Design review of the part built by this model. Coordinates are the model's own, in mm. Face numbers are marked on the shaded views. A direction names the side the tool comes from. Coordinates: 2 decimals unless noted, no trailing zeros. Write each loop counter-clockwise with the first axis right and the second up, starting at its lowest first coordinate (ties: lowest second). Pieces come first, ordered by that corner, then holes. Notation, with made-up numbers: M -16,-13 L 22,-13 A24 ccw 22,-3 Z; hole C 84.5,-9 d9. An arc over 180 degrees is marked long. One line per question, with ' | ' between items.
from build123d import *

# Parameters (mm, degrees)
F1_DEPTH = 2.8
F2_R     = 0.55
F3_DEPTH = 5
F4_R     = 1
F5_R     = 0.3
F7_W     = 2.5907744158
F7_H     = 2.3
F8_DEPTH = 1.5
F9_R     = 0.5


with BuildPart() as f1:
    # F0 (on Top) → F1 (new body)
    with BuildSketch(Plane.XY):
        with BuildLine():
            Line((-4.2, -2.5), (-3.2, -2.5))
            Line((-3.2, -2.5), (-3.2, -1.9))
            ThreePointArc((-3.2, -1.9), (-2.9071067812, -1.1928932188), (-2.2, -0.9))
            Line((-2.2, -0.9), (0, -0.9))
            Line((0, -0.9), (0, -2.3))
            Line((0, -2.3), (1.8, -2.3))
            Line((1.8, -2.3), (1.8, -1.3))
            Line((1.8, -1.3), (5.2, -1.3))
            Line((5.2, -1.3), (5.2, 0))
            Line((5.2, 0), (5.2, 1.3))
            Line((5.2, 1.3), (1.8, 1.3))
            Line((1.8, 1.3), (1.8, 2.3))
            Line((1.8, 2.3), (0, 2.3))
            Line((0, 2.3), (0, 0.9))
            Line((0, 0.9), (-2.2, 0.9))
            ThreePointArc((-2.2, 0.9), (-2.9071067812, 1.1928932188), (-3.2, 1.9))
            Line((-3.2, 1.9), (-3.2, 2.5))
            Line((-3.2, 2.5), (-4.2, 2.5))
            Line((-4.2, 2.5), (-4.6408174518, 0))
            Line((-4.6408174518, 0), (-4.2, -2.5))
        make_face()
    extrude(amount=F1_DEPTH)

    # F2 (on face) → F3 (join)
    with BuildSketch(Plane(origin=(0, 0, 0), x_dir=(1, 0, 0), z_dir=(0, 0, -1))):
        with BuildLine():
            Line((-4.2, -2.5), (-3.2, -2.5))
            Line((-3.2, -2.5), (-3.2, -1.9))
            ThreePointArc((-3.2, -1.9), (-2.9071067812, -1.1928932188), (-2.2, -0.9))
            Line((-2.2, -0.9), (-2.2, 0.9))
            ThreePointArc((-2.2, 0.9), (-2.9071067812, 1.1928932188), (-3.2, 1.9))
            Line((-3.2, 1.9), (-3.2, 2.5))
            Line((-3.2, 2.5), (-4.2, 2.5))
            Line((-4.2, 2.5), (-4.6408174518, 0))
            Line((-4.6408174518, 0), (-4.2, -2.5))
        make_face()
        with Locations((-3.6, 0)):
            Circle(F2_R, mode=Mode.SUBTRACT)
    extrude(amount=F3_DEPTH)

    # F4
    f4_edges = [f1.edges().sort_by_distance(p)[0] for p in [
        (-2.2, 0, 0),
        (-4.640817, 0, -1.1),
    ]]
    fillet(f4_edges, radius=F4_R)

    # F5
    f5_edges = [f1.edges().sort_by_distance(p)[0] for p in [
        (5.2, -1.3, 1.4),
        (5.2, 1.3, 1.4),
        (-3.2, 2.5, -1.1),
        (-4.2, 2.5, -1.1),
        (-3.2, -2.5, -1.1),
        (-4.2, -2.5, -1.1),
        (-0.6, 0.9, 0),
        (-1.2, 0, 0),
        (0, 1.6, 0),
        (-0.6, -0.9, 0),
        (0.9, 2.3, 0),
        (0, -1.6, 0),
        (1.8, 1.8, 0),
        (0.9, -2.3, 0),
        (3.5, 1.3, 0),
        (1.8, -1.8, 0),
        (5.2, 0, 0),
        (3.5, -1.3, 0),
    ]]
    fillet(f5_edges, radius=F5_R)

    # F7 (on offset) → F8 (cut)
    with BuildSketch(Plane.XY.offset(-3.2)):
        with Locations((-3.6953872079, 0)):
            Rectangle(F7_W, F7_H)
    extrude(amount=F8_DEPTH, mode=Mode.SUBTRACT)

    # F9
    f9_edges = [f1.edges().sort_by_distance(p)[0] for p in [
        (-4.438041, 1.15, -2.45),
        (-4.438041, -1.15, -2.45),
    ]]
    fillet(f9_edges, radius=F9_R)


solid = f1.part
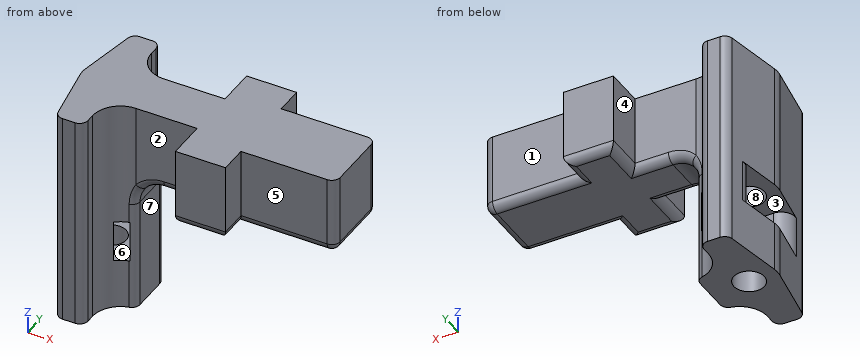
1. Take a section at D-D (z = -2). Write out the cut boundary in (x, y), then the cut area to 3 significant figures.
Answer sheet:
outline: M -4.33,-1.74 L -4.24,-2.25 A0.3 ccw -3.95,-2.5 L -3.5,-2.5 A0.3 ccw -3.2,-2.2 L -3.2,-1.9 A1 cw -2.86,-1.15 L -3.84,-1.15 A0.5 ccw Z; M -4.33,1.74 A0.5 ccw -3.84,1.15 L -2.86,1.15 A1 cw -3.2,1.9 L -3.2,2.2 A0.3 ccw -3.5,2.5 L -3.95,2.5 A0.3 ccw -4.24,2.25 Z; M -2.4,-0.92 A0.3 ccw -2.2,-0.64 L -2.2,0.64 A0.3 ccw -2.4,0.92 Z | area: 3.29 mm^2
2. Insertion check: pin 1 Ø1.2 at (x, z) = (2.5, 1) entering from -Y; pin 2 Ø0.7 at (x, z) = (-1, 1.5) entering from +Y; pin 3 Ø0.5 at (x, z) = (0.5, 1.5) entering from -Y. Each pin has a flat end and moves straight along its axis. Give the tip position at first contact, or say it passes through.
Answer sheet:
pin 1: y = -1.3 | pin 2: y = 0.9 | pin 3: y = -2.3
3. Draft analysis for pull direction X (two halves, no side actions). For the marked faces 6, 7 and 8, state which applies: pulls with the +X half, pulls with the -X half, needs draft (parallel to the pull), parting line crosses it, or undercut.
Answer sheet:
face 6: needs draft | face 7: pulls with the +X half | face 8: undercut
4. Take a section at A-A (y = 0). Write out the cut boundary in (x, z), then the cut area to 3 significant figures.
Answer sheet:
outline: M -4.63,-5 L -4.15,-5 L -4.15,-3.2 L -4.63,-3.2 Z; M -4.63,-1.7 L -4.15,-1.7 L -4.15,0 L -3.05,0 L -3.05,-1.7 L -2.4,-1.7 L -2.4,-3.2 L -3.05,-3.2 L -3.05,-5 L -2.2,-5 L -2.2,-1 A1 cw -1.2,0 L 4.9,0 A0.3 ccw 5.2,0.3 L 5.2,2.8 L -4.63,2.8 Z | area: 32.6 mm^2
5. Tool access review of the marked faces 1, 2, 3, 4 and 5: name each direction out of +Z, -Z, +X, -X, +Y, -Y from which nothing blocks a thin tool from reaching the whole face with its end or side.
Answer sheet:
face 1: +Z, -Z, +X, +Y | face 2: +Z, -Z, -Y | face 3: -X | face 4: +Z, -Z, +Y | face 5: +Z, -Z, +X, -Y
6. Take a section at C-C (z = 2). Write out the cut boundary in (x, y), then the cut area to 3 significant figures.
Answer sheet:
outline: M -4.61,-0.17 L -4.24,-2.25 A0.3 ccw -3.95,-2.5 L -3.5,-2.5 A0.3 ccw -3.2,-2.2 L -3.2,-1.9 A1 cw -2.2,-0.9 L 0,-0.9 L 0,-2.3 L 1.8,-2.3 L 1.8,-1.3 L 4.9,-1.3 A0.3 ccw 5.2,-1 L 5.2,1 A0.3 ccw 4.9,1.3 L 1.8,1.3 L 1.8,2.3 L 0,2.3 L 0,0.9 L -2.2,0.9 A1 cw -3.2,1.9 L -3.2,2.2 A0.3 ccw -3.5,2.5 L -3.95,2.5 A0.3 ccw -4.24,2.25 L -4.61,0.17 A1 ccw Z | area: 29.3 mm^2
7. Take a section at B-B (x = -1). Write out the cut boundary in (y, z).
Answer sheet:
outline: M -0.9,0.3 A0.3 ccw -0.6,0 L 0.6,0 A0.3 ccw 0.9,0.3 L 0.9,2.8 L -0.9,2.8 Z
8. To check wall thickness, follow line 1 along X through (y, z) = (0, -3.7); line 2 along Y through (x, z) = (-3.6, -0.4); line 3 along Z through (x, y) = (3.25, 0.9). State the ranges of each line that lie inside material, in increasing order. Write a range as [from, to].
Answer sheet:
line 1: [-4.63, -4.15], [-3.05, -2.2] | line 2: [-2.5, -0.55], [0.55, 2.5] | line 3: [0, 2.8]
